```python
from build123d import *

# Parameters (mm, degrees)
EXTRUDE_START               = -28
EXTRUDE_1_DEPTH             = 38
EXTRUDE_2_DEPTH             = 16
EXTRUDE_3_DEPTH             = 18
EXTRUDE_4_DEPTH             = 2
CUT_EXTRUDE_1_DEPTH         = 20
SKETCH_6_W                  = 16
SKETCH_6_H                  = 22
CUT_EXTRUDE_2_DEPTH         = 2
SKETCH_7_W                  = 2
SKETCH_7_H                  = 22
CUT_EXTRUDE_3_DEPTH         = 16
SKETCH_8_W                  = 16
SKETCH_8_H                  = 22
CUT_EXTRUDE_4_DEPTH         = 16
CUT_EXTRUDE_5_DEPTH         = 18
CUT_EXTRUDE_6_DEPTH         = 16
SKETCH_11_W                 = 16
SKETCH_11_H                 = 22
CUT_EXTRUDE_7_DEPTH         = 16
CUT_EXTRUDE_8_DEPTH         = 20
CUT_EXTRUDE_START           = -16
CUT_EXTRUDE_9_DEPTH         = 16
CUT_EXTRUDE_10_DEPTH        = 16
CUT_EXTRUDE_11_DEPTH        = 20
EXTRUDE_START_2             = 2
EXTRUDE_5_DEPTH             = 2
HOLE_WIZARD_11_0_11_1_D     = 11
HOLE_WIZARD_11_0_11_1_DEPTH = 32
HOLE_WIZARD_8_0_8_1_D       = 8
HOLE_WIZARD_8_0_8_1_DEPTH   = 2
HOLE_WIZARD_2_0_2_1_D       = 2
HOLE_WIZARD_2_0_2_1_DEPTH   = 2
HOLE_WIZARD_8_0_8_2_D       = 8
HOLE_WIZARD_8_0_8_2_DEPTH   = 56
HOLE_WIZARD_2_0_2_2_D       = 2
HOLE_WIZARD_2_0_2_2_DEPTH   = 56
HOLE_WIZARD_8_0_8_3_D       = 8
HOLE_WIZARD_8_0_8_3_DEPTH   = 2
HOLE_WIZARD_2_0_2_3_D       = 2
HOLE_WIZARD_2_0_2_3_DEPTH   = 2
HOLE_WIZARD_8_0_8_4_D       = 8
HOLE_WIZARD_2_0_2_4_D       = 2
FILLET_1_R                  = 0.5
FILLET_2_R                  = 2
FILLET_3_R                  = 2.5
FILLET_4_R                  = 10


with BuildPart() as part:
    # 凸台-拉伸1: read off the stored shape, not the designer's step
    # 凸台-拉伸1 outline → 凸台-拉伸1 (new body)
    with BuildSketch(Plane.XY.offset(EXTRUDE_START)):
        with BuildLine():
            Line((10, -20), (10, 22))
            ThreePointArc((10, 22), (0, 32), (-10, 22))
            Line((-10, 22), (-26, 22))
            Line((-26, 22), (-26, -20))
            Line((-26, -20), (10, -20))
        make_face()
    extrude(amount=EXTRUDE_1_DEPTH)

    # 草图2 → 凸台-拉伸2 (add)
    with BuildSketch(Plane.XY.offset(10)):
        with BuildLine():
            Line((10, 22), (10, -20))
            Line((10, -20), (-26, -20))
            Line((-26, -20), (-26, 22))
            Line((-26, 22), (-10, 22))
            ThreePointArc((-10, 22), (0, 32), (10, 22))
        make_face()
    extrude(amount=EXTRUDE_2_DEPTH)

    # 草图3 → 凸台-拉伸3 (add)
    with BuildSketch(Plane(origin=(10, 0, 0), x_dir=(0, 0, -1), z_dir=(1, 0, 0))):
        with BuildLine():
            Line((-10, -20), (-10, 22))
            Line((-10, 22), (10, 22))
            Line((10, 22), (26, 22))
            Line((26, 22), (28, 22))
            Line((28, 22), (28, -20))
            Line((28, -20), (10, -20))
            ThreePointArc((10, -20), (0, -30), (-10, -20))
        make_face()
    extrude(amount=EXTRUDE_3_DEPTH)

    # 草图4 → 凸台-拉伸4 (add)
    with BuildSketch(Plane.XY.offset(26)):
        with BuildLine():
            Line((10, 22), (10, -20))
            Line((10, -20), (-26, -20))
            Line((-26, -20), (-26, 22))
            Line((-26, 22), (-10, 22))
            ThreePointArc((-10, 22), (0, 32), (10, 22))
        make_face()
    extrude(amount=EXTRUDE_4_DEPTH)

    # 草图5 → 切除-拉伸1 (cut)
    with BuildSketch(Plane.XZ.offset(20)):
        Polygon((-26, 28), (-26, -28), (28, -28), (28, -10), (10, -10), (10, 10), (10, 28), align=None)
    extrude(amount=-CUT_EXTRUDE_1_DEPTH, mode=Mode.SUBTRACT)

    # 草图6 → 切除-拉伸2 (cut)
    with BuildSketch(Plane(origin=(0, 0, -28), x_dir=(-1, 0, 0), z_dir=(0, 0, -1))):
        with Locations((18, 11)):
            Rectangle(SKETCH_6_W, SKETCH_6_H)
    extrude(amount=-CUT_EXTRUDE_2_DEPTH, mode=Mode.SUBTRACT)

    # 草图7 → 切除-拉伸3 (cut)
    with BuildSketch(Plane.ZY.offset(26)):
        with Locations((27, 11)):
            Rectangle(SKETCH_7_W, SKETCH_7_H)
    extrude(amount=-CUT_EXTRUDE_3_DEPTH, mode=Mode.SUBTRACT)

    # 草图8 → 切除-拉伸4 (cut)
    with BuildSketch(Plane(origin=(0, 0, -26), x_dir=(-1, 0, 0), z_dir=(0, 0, -1))):
        with Locations((18, 11)):
            Rectangle(SKETCH_8_W, SKETCH_8_H)
    extrude(amount=-CUT_EXTRUDE_4_DEPTH, mode=Mode.SUBTRACT)

    # 草图9 → 切除-拉伸5 (cut)
    with BuildSketch(Plane(origin=(28, 0, 0), x_dir=(0, 0, -1), z_dir=(1, 0, 0))):
        Polygon((28, 22), (26, 22), (10, 22), (10, 0), (28, 0), align=None)
    extrude(amount=-CUT_EXTRUDE_5_DEPTH, mode=Mode.SUBTRACT)

    # 草图10 → 切除-拉伸6 (cut)
    with BuildSketch(Plane.ZY.offset(-10)):
        with BuildLine():
            Line((-10, 0), (-10, -20))
            ThreePointArc((-10, -20), (0, -30), (10, -20))
            Line((10, -20), (10, 0))
            Line((10, 0), (-10, 0))
        make_face()
    extrude(amount=-CUT_EXTRUDE_6_DEPTH, mode=Mode.SUBTRACT)

    # 草图11 → 切除-拉伸7 (cut)
    with BuildSketch(Plane.XY.offset(26)):
        with Locations((-18, 11)):
            Rectangle(SKETCH_11_W, SKETCH_11_H)
    extrude(amount=-CUT_EXTRUDE_7_DEPTH, mode=Mode.SUBTRACT)

    # 草图12 → 切除-拉伸8 (cut)
    with BuildSketch(Plane(origin=(0, 0, -10), x_dir=(-1, 0, 0), z_dir=(0, 0, -1))):
        with BuildLine():
            Line((-10, 22), (10, 22))
            ThreePointArc((10, 22), (0, 32), (-10, 22))
        make_face()
    extrude(amount=-CUT_EXTRUDE_8_DEPTH, mode=Mode.SUBTRACT)

    # 草图13 → 切除-拉伸9 (cut)
    with BuildSketch(Plane.XY.offset(-10).offset(CUT_EXTRUDE_START)):
        with BuildLine():
            Line((-10, 22), (10, 22))
            ThreePointArc((10, 22), (0, 32), (-10, 22))
        make_face()
    extrude(amount=CUT_EXTRUDE_9_DEPTH, mode=Mode.SUBTRACT)

    # 草图14 → 切除-拉伸10 (cut)
    with BuildSketch(Plane(origin=(0, 0, 10), x_dir=(-1, 0, 0), z_dir=(0, 0, -1))):
        with BuildLine():
            Line((-10, 22), (10, 22))
            ThreePointArc((10, 22), (0, 32), (-10, 22))
        make_face()
    extrude(amount=-CUT_EXTRUDE_10_DEPTH, mode=Mode.SUBTRACT)

    # 草图15 → 切除-拉伸11 (cut)
    with BuildSketch(Plane(origin=(0, 22, 0), x_dir=(-1, 0, 0), z_dir=(0, 1, 0))):
        Polygon((26, -10), (26, 10), (10, 10), (10, 26), (-10, 26), (-10, 10), (-28, 10), (-28, -10), (-10, -10), (-10, -26), (10, -26), (10, -10), align=None)
    extrude(amount=-CUT_EXTRUDE_11_DEPTH, mode=Mode.SUBTRACT)

    # 草图16 → 凸台-拉伸5 (add)
    with BuildSketch(Plane.ZY.offset(26).offset(EXTRUDE_START_2)):
        with BuildLine():
            Line((10, 2), (10, -20))
            ThreePointArc((10, -20), (0, -30), (-10, -20))
            Line((-10, -20), (-10, 2))
            Line((-10, 2), (10, 2))
        make_face()
    extrude(amount=-EXTRUDE_5_DEPTH)

    # Ø11.0 (11) 直径孔1
    with Locations(Plane(origin=(0, 0, 0), x_dir=(-1, 0, 0), z_dir=(0, -1, 0))):
        with Locations((0, 0)):
            Hole(HOLE_WIZARD_11_0_11_1_D / 2, depth=HOLE_WIZARD_11_0_11_1_DEPTH)

    # Ø8.0 (8) 直径孔1
    with Locations(Plane.XY.offset(28)):
        with Locations((0, 22)):
            Hole(HOLE_WIZARD_8_0_8_1_D / 2, depth=HOLE_WIZARD_8_0_8_1_DEPTH)

    # Ø2.0 (2) 直径孔1
    with Locations(Plane.XY.offset(28)):
        with Locations((0, 15), (7, 22), (-7, 22), (0, 29)):
            Hole(HOLE_WIZARD_2_0_2_1_D / 2, depth=HOLE_WIZARD_2_0_2_1_DEPTH)

    # Ø8.0 (8) 直径孔2
    with Locations(Plane(origin=(0, 0, -28), x_dir=(-1, 0, 0), z_dir=(0, 0, -1))):
        with Locations((0, 22)):
            Hole(HOLE_WIZARD_8_0_8_2_D / 2, depth=HOLE_WIZARD_8_0_8_2_DEPTH)

    # Ø2.0 (2) 直径孔2
    with Locations(Plane(origin=(0, 0, -28), x_dir=(-1, 0, 0), z_dir=(0, 0, -1))):
        with Locations((0, 15), (-7, 22), (7, 22), (0, 29)):
            Hole(HOLE_WIZARD_2_0_2_2_D / 2, depth=HOLE_WIZARD_2_0_2_2_DEPTH)

    # Ø8.0 (8) 直径孔3
    with Locations(Plane(origin=(-26, 0, 0), x_dir=(0, 0, -1), z_dir=(1, 0, 0))):
        with Locations((0, -20)):
            Hole(HOLE_WIZARD_8_0_8_3_D / 2, depth=HOLE_WIZARD_8_0_8_3_DEPTH)

    # Ø2.0 (2) 直径孔3
    with Locations(Plane(origin=(-26, 0, 0), x_dir=(0, 0, -1), z_dir=(1, 0, 0))):
        with Locations((0, -13), (0, -27), (7, -20), (-7, -20)):
            Hole(HOLE_WIZARD_2_0_2_3_D / 2, depth=HOLE_WIZARD_2_0_2_3_DEPTH)

    # Ø8.0 (8) 直径孔4 (through all)
    with Locations(Plane.ZY.offset(-26)):
        with Locations((0, -20)):
            Hole(HOLE_WIZARD_8_0_8_4_D / 2)

    # Ø2.0 (2) 直径孔4 (through all)
    with Locations(Plane.ZY.offset(-26)):
        with Locations((0, -13), (0, -27), (-7, -20), (7, -20)):
            Hole(HOLE_WIZARD_2_0_2_4_D / 2)

    # 圆角1
    fillet_1_edges = [part.edges().sort_by_distance(p)[0] for p in [
        (26, 0, 0),
        (-26, 0, 0),
    ]]
    fillet(fillet_1_edges, radius=FILLET_1_R)

    # 圆角2
    fillet_2_edges = [part.edges().sort_by_distance(p)[0] for p in [
        (0, 0, 28),
        (0, 0, -28),
    ]]
    fillet(fillet_2_edges, radius=FILLET_2_R)

    # 圆角3
    fillet_3_edges = [part.edges().sort_by_distance(p)[0] for p in [
        (28, 2, 0),
        (-28, 2, 0),
    ]]
    fillet(fillet_3_edges, radius=FILLET_3_R)

    # 圆角4
    fillet_4_edges = [part.edges().sort_by_distance(p)[0] for p in [
        (-10, 1, 10),
        (10, 1, -10),
        (-10, 1, -10),
        (10, 1, 10),
    ]]
    fillet(fillet_4_edges, radius=FILLET_4_R)


solid = part.part
```
The listing builds one solid part. Answer for the finished solid, in the listing's coordinates (mm). A direction names the side the tool comes from. Coordinates: 2 decimals unless noted, no trailing zeros. Write each loop counter-clockwise with the first axis right and the second up, starting at its lowest first coordinate (ties: lowest second). Pieces come first, ordered by that corner, then holes. Notation, with made-up numbers: (10, 1) - (49, 1) arc R20 ccw to (49, 19) - close; hole circle Ø7 at (-9.75, 34). An arc over 180 degrees is marked (long way). Return JSON: item names as keys, results as strings. Group by question number.
Q1. Flat-ended cylindrical pins translate along their axes: pin 1 Ø4 at (y, z) = (7, -25.5) entering from -X; pin 2 Ø6 at (x, z) = (-17, -2.5) entering from +Y; pin 3 Ø5 at (y, z) = (1, -19) entering from -X. Find the tip coordinate at first contact, or state that the pin passes through.
Q2. The part is cut by section D-D on z = -7. Write down the section's boundary in (x, y), and give its area (3 significant figures).
Q3. Which of the six approach directions +Z, -Z, +X, -X, +Y, -Y give full straight-line access (tool end or side, diameter ignored) to faces 5 (the cylindrical face through (0, 32, 27)), 6 (the flat face through (-26.4, -7.3, 10)), 7 (the flat face through (0, 17, -26)), 8 (the flat face through (26.4, -7.3, -10))?
Q4. For a pull along X with two mould halves and no side action, classify faces 1 (the cylindrical face through (-13.01, 1.01, 12.85)), 2 (the cylindrical face through (0, 30, -27)), 3 (the cylindrical face through (27, -21, 7)), 4 (the cylindrical face through (-7, 21, 27)) as +X half, -X half, draft (parallel to the pull), parting line (faces both ways), or undercut.
Q5. The part is cut by section A-A on x = -7. Write down the section's boundary in (y, z).
Q6. Find the intervals of material crossed by line 1 along Z through (x, y) = (-26.6, -20); line 2 along Y through (x, z) = (-27.6, 0); line 3 along Y through (x, z) = (-9.5, 17.5), in increasing order. Write a range as [from, to].
Q7. The part is cut by section B-B on y = -27. Write down the section's boundary in (x, z), and give its area (3 significant figures).
Q8. The part is cut by section C-C on y = -6.5. Write down the section's boundary in (x, z).
Evaluation:
{
 "1": {"pin 1": "stops at x = -10", "pin 2": "stops at y = 2", "pin 3": "stops at x = -10.63"},
 "2": {"outline": "(-28, -27.14) - (-26, -27.14) - (-26, -21) - (-28, -21) - close; (-28, -19) - (-26, -19) - (-26, -0.5) arc R0.5 cw to (-25.5, 0) - (25.5, 0) arc R0.5 cw to (26, -0.5) - (26, -19) - (28, -19) - (28, -0.5) arc R2.5 ccw to (25.5, 2) - (-25.5, 2) arc R2.5 ccw to (-28, -0.5) - close; (26, -27.14) - (28, -27.14) - (28, -21) - (26, -21) - close", "area": "210 mm2"},
 "3": {"face 5": "+Z, -Z, +Y", "face 6": "+Z, -X, +Y, -Y", "face 7": "+X, -X, +Y", "face 8": "-Z, +X, +Y, -Y"},
 "4": {"face 1": "-X half", "face 2": "undercut", "face 3": "draft", "face 4": "undercut"},
 "5": {"outline": "(0, -26) arc R2 ccw to (2, -28) - (21, -28) - (21, -26) - (2, -26) - (2, 26) - (21, 26) - (21, 28) - (2, 28) arc R2 ccw to (0, 26) - close; (23, -28) - (29.14, -28) - (29.14, -26) - (23, -26) - close; (23, 26) - (29.14, 26) - (29.14, 28) - (23, 28) - close"},
 "6": {"line 1": "z = [-10, -8], [-6, -4], [4, 6], [8, 10]", "line 2": "y = [-30, -28], [-26, -24], [-16, -14], [-12, 0.86]", "line 3": "y = [0, 2]"},
 "7": {"outline": "(-28, -7.14) - (-26, -7.14) - (-26, -1) - (-28, -1) - close; (-28, 1) - (-26, 1) - (-26, 7.14) - (-28, 7.14) - close; (26, -7.14) - (28, -7.14) - (28, -1) - (26, -1) - close; (26, 1) - (28, 1) - (28, 7.14) - (26, 7.14) - close", "area": "49.1 mm2"},
 "8": {"outline": "(-28, -10) - (-26, -10) - (-26, 10) - (-28, 10) - close; (26, -10) - (28, -10) - (28, 10) - (26, 10) - close"}
}
